Geometry check sheet. Reference: the model listing, model coordinates, mm. A direction names the side the tool comes from. Give positions to 0.01 mm unless a question says otherwise; leave off trailing zeros. Order: outer loops, then holes, each group sorted by start corner. A loop starts at its lowest first (then second) coordinate and runs counter-clockwise, first axis right, second up. Notation, with made-up numbers: M 31.5,-8 L 69.5,-8 A25 cw 69.5,4 Z; hole C 50,-2.75 d8. An arc over 180 degrees is marked long. Answer as CSV lines item,"result". Start each with the question number.
```python
from build123d import *

# Parameters (mm, degrees)
F0_W     = 30
F0_H     = 20
F0_H_2   = 100
F1_DEPTH = 2.5
F2_DEPTH = 30
F3_R     = 14.99999


# Not quite as in the source:
# - a fillet or chamfer is up to 0.001 mm smaller than in the source, because OpenCascade refuses the exact size


with BuildPart() as f1:
    # F0 (on Top) → F1 (new body, symmetric)
    with BuildSketch(Plane.XY):
        with BuildLine():
            Line((-30, 10), (-30, 30))
            Line((-30, 30), (-250.9035135708, 9.9590995189))
            ThreePointArc((-250.9035135708, 9.9590995189), (-243.2559335601, 7.3836012794), (-240, 0))
            ThreePointArc((-240, 0), (-244.5708205421, -8.3978574895), (-254.1048020827, -9.1186950745))
            Line((-254.1048020827, -9.1186950745), (-30, -110))
            Line((-30, -110), (-30, -90))
            Line((-30, -90), (-30, 10))
        make_face()
        with BuildLine():
            ThreePointArc((-50.9035135708, 8.1035827434), (-43.2559335601, 5.5280845039), (-40, -1.8555167755))
            Line((-40, -1.8555167755), (-40, -70.0304714473))
            ThreePointArc((-40, -70.0304714473), (-44.5708205421, -78.4283289367), (-54.1048020827, -79.1491665218))
            Line((-54.1048020827, -79.1491665218), (-180.1505302804, -22.409384854))
            ThreePointArc((-180.1505302804, -22.409384854), (-185.9078460259, -11.6358085325), (-176.9492417684, -3.3315902606))
            Line((-176.9492417684, -3.3315902606), (-50.9035135708, 8.1035827434))
        make_face(mode=Mode.SUBTRACT)
        with BuildLine():
            ThreePointArc((-240, 0), (-243.2559335601, 7.3836012794), (-250.9035135708, 9.9590995189))
            ThreePointArc((-250.9035135708, 9.9590995189), (-259.8621178282, 1.654881247), (-254.1048020827, -9.1186950745))
            ThreePointArc((-254.1048020827, -9.1186950745), (-244.5708205421, -8.3978574895), (-240, 0))
        make_face()
        with Locations((-15, 20)):
            Rectangle(F0_W, F0_H)
        with Locations((-15, -40)):
            Rectangle(F0_W, F0_H_2)
        with Locations((-15, -100)):
            Rectangle(F0_W, F0_H)
    extrude(amount=F1_DEPTH, both=True)

    # F0 (on Top) → F2 (join)
    with BuildSketch(Plane.XY):
        with Locations((-15, 20)):
            Rectangle(F0_W, F0_H)
        with Locations((-15, -100)):
            Rectangle(F0_W, F0_H)
    extrude(amount=F2_DEPTH)

    # F3 (radius 15 in the source; OpenCascade refuses exactly that, so slightly less here)
    f3_edges = [f1.edges().sort_by_distance(p)[0] for p in [
        (0, 20, 30),
        (-30, 20, 30),
        (0, -100, 30),
        (-30, -100, 30),
    ]]
    fillet(f3_edges, radius=F3_R)


solid = f1.part
```
Item 1: Depth check by flat-ended pin: pin 1 Ø4 at (y, z) = (15, 11.5) entering from -X; pin 2 Ø6 at (x, y) = (-180.5, 1) entering from +Z; pin 3 Ø1.5 at (x, z) = (-34.5, 1.5) entering from -Y. Enter the tip coordinate at first touch or a pass-through.
Item 2: Section check B-B on y = -12.5. Record the boundary of the cut face in (x, z), then the cut area to 3 significant figures.
Item 3: Draft check along X on faces 1 (the face through (-114.809, 2.306, 0.035)), 2 (the face through (-103, 8, -2.5)), 3 (the face through (-4.51, 20.14, 25.72)). Enter one of: pulls with the +X half, pulls with the -X half, needs draft (parallel to the pull), parting line crosses it, or undercut.
Item 4: Section check D-D on x = -233. Record the boundary of the cut face in (y, z), then the cut area to 3 significant figures.
Item 5: Access from +Z, -Z, +X, -X, +Y, -Y to the whole of each face (thin tool, end or side, straight path). Record for faces 4 (the face through (-30, 20, 9)), 5 (the face through (-43.342, 5.606, 0.035)), 6 (the face through (-259.83, 1.84, 0.04)), 7 (the face through (-15, -90, 16)).
Item 6: Scan lines: line 1 along Y through (x, z) = (-23, 13); line 2 along Z through (x, y) = (-172, -36); line 3 along X through (y, z) = (24, 11). Record each from-to range of solid material in increasing order.
Item 7: Section check A-A on z = 8. Record the boundary of the cut face in (x, y).
Numbers:
1,pin 1,"x = -30"
1,pin 2,"z = 2.5"
1,pin 3,"y = -108.31"
2,outline,"M -246.59,-2.5 L -186.01,-2.5 L -186.01,2.5 L -246.59,2.5 Z; M -40,-2.5 L 0,-2.5 L 0,2.5 L -40,2.5 Z"
2,area,"503 mm2"
3,face 1,"undercut"
3,face 2,"needs draft"
3,face 3,"pulls with the +X half"
4,outline,"M -18.62,-2.5 L 11.58,-2.5 L 11.58,2.5 L -18.62,2.5 Z"
4,area,"151 mm2"
5,face 4,"+Z, -X, +Y, -Y"
5,face 5,"+Z, -Z"
5,face 6,"+Z, -Z, -X"
5,face 7,"+Z, +X, -X"
6,line 1,"-110 to -90, 10 to 30"
6,line 2,"-2.5 to 2.5"
6,line 3,"-30 to 0"
7,outline,"M -30,-110 L 0,-110 L 0,-90 L -30,-90 Z; M -30,10 L 0,10 L 0,30 L -30,30 Z"
